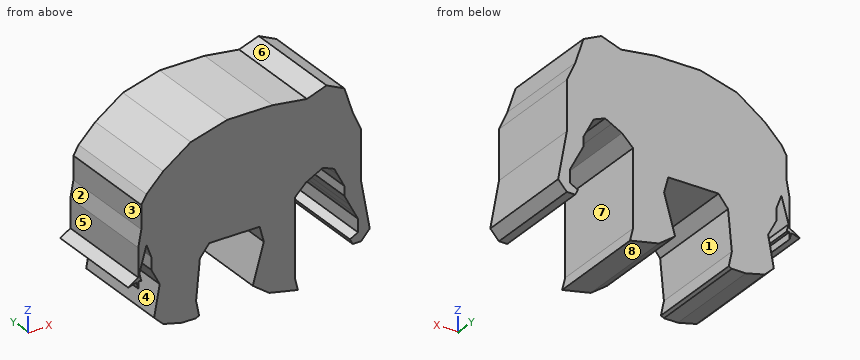
```python
from build123d import *

# Parameters (mm, degrees)
F1_DEPTH = 25.4


with BuildPart() as f1:
    # F0 (on Front) → F1 (new body)
    with BuildSketch(Plane.XZ):
        Polygon((19.687949, 25.243243), (14.781063, 23.544706), (6.194014, 24.701377), (-5.051399, 24.701377), (-14.188432, 22.223622), (-21.076944, 17.4111), (-25.228923, 13.259119), (-26.514801, 11.088767), (-26.514801, 5.281893), (-27.283788, 1.180633), (-27.283788, -5.896606), (-29.806441, -7.50078), (-27.718788, -6.934656), (-27.283788, -8.538775), (-27.283788, -6.790471), (-26.514801, -6.934656), (-27.021825, -5.06494), (-25.228923, 1.180633), (-24.035911, -2.027715), (-24.035911, -5.06494), (-21.926213, -9.104954), (-23.341661, -16.654009), (-21.076944, -18.824359), (-16.358785, -19.973479), (-12.867347, -19.973479), (-12.112442, -19.579267), (-12.867347, -15.899101), (-11.923715, -6.085332), (-9.564636, -3.160073), (2.985667, -3.160073), (4.023661, -7.028964), (1.287129, -16.654009), (5.344746, -19.579267), (12.516348, -21.089077), (11.761442, -17.975092), (11.761442, -16.654009), (11.761442, 1.08627), (14.527172, 3.790959), (17.145273, 5.158133), (18.744318, 5.993155), (21.584706, 4.860796), (22.52096, 3.067896), (24.123017, 0), (24.123017, -2.335592), (25.511982, -4.995424), (26.670383, -7.213729), (27.510151, -8.821864), (27.510151, -12.030212), (25.511982, -13.073657), (26.199007, -14.389291), (28.275, -14.389291), (30.445352, -12.030212), (28.275, 0), (28.275, 1.841175), (28.275, 4.860796), (28.275, 12.221124), (26.199007, 16.844919), (24.123017, 23.167253), align=None)
    extrude(amount=F1_DEPTH)


solid = f1.part
```
Geometry check sheet. Reference: the model listing, model coordinates, mm. Face numbers are marked on the shaded views. A direction names the side the tool comes from. Round coordinates to 2 decimals unless told otherwise and drop trailing zeros. Loops run counter-clockwise (first coordinate to the right, second up) from the corner with the lowest first, then second, coordinate; pieces in that order, holes last. Notation, with made-up numbers: (40.25, 42) - (47.25, 42) arc R29 ccw to (47.25, 62) - close; hole circle Ø3 at (8, 15). An arc over 180 degrees is marked (long way). Write item = value, one per line. Start each with the question number.
1. Section check C-C on x = -6. Enter the section's corners in (y, z), then the cut area to 3 significant figures.
2. Depth check by flat-ended pin: pin 1 (14 mm diameter, centred on x = -5.5, y = -11, fed in from -Z); pin 2 (10 mm diameter, centred on x = 16, y = -5, fed in from -Z); pin 3 (0.7 mm diameter, centred on y = -13.5, z = -1.5, fed in from -X). Enter the tip coordinate at first touch or a pass-through.
3. Section check A-A on z = -4. Enter the section's corners in (x, y), then the cut area to 3 significant figures.
4. Thickness scan on line 1 (X direction, y = -19, z = -10); line 2 (X direction, y = -11, z = -9); line 3 (X direction, y = -20.25, z = -6). Record the ranges inside material, lowest first.
5. Set-up check for the marked faces 4, 5, 6, 7 and 8: record each of +Z, -Z, +X, -X, +Y, -Y from which the full face is reachable in a straight line by a thin tool's end or side.
6. Mould release check, pull along Z, two halves, no side actions. Record for the marked faces 1, 2 and 3: released by +Z, released by -Z, zero draft, split by the parting line, or undercut.
7. Section check B-B on z = 2. Enter the section's corners in (x, y) (3 decimals).
8. Section check D-D on x = 7.5. Enter the section's corners in (y, z).
Working result:
q1.outline = (-25.4, -3.16) - (0, -3.16) - (0, 24.44) - (-25.4, 24.44) - close
q1.area = 701 mm^2
q2.pin_1 = -19.78
q2.pin_2 = -21.09
q2.pin_3 = -27.28
q3.outline = (-27.28, -25.4) - (-26.72, -25.4) - (-26.72, 0) - (-27.28, 0) - close; (-24.04, -25.4) - (-10.24, -25.4) - (-10.24, 0) - (-24.04, 0) - close; (3.21, -25.4) - (11.76, -25.4) - (11.76, 0) - (3.21, 0) - close; (24.99, -25.4) - (29, -25.4) - (29, 0) - (24.99, 0) - close
q3.area = 684 mm^2
q4.line_1 = -22.09 to -12.3, 3.18 to 11.76, 27.51 to 30.08
q4.line_2 = -21.98 to -12.2, 3.46 to 11.76, 27.51 to 29.9
q4.line_3 = -27.45 to -26.77, -23.55 to -11.85, 3.75 to 11.76, 26.04 to 29.36
q5.face_4 = -X, +Y, -Y
q5.face_5 = +Z, -X, +Y, -Y
q5.face_6 = +Z, +Y, -Y
q5.face_7 = +Y, -Y
q5.face_8 = -Z, +Y, -Y
q6.face_1 = undercut
q6.face_2 = released by +Z
q6.face_3 = zero draft
q7.outline = (-27.13, -25.4) - (12.696, -25.4) - (12.696, 0) - (-27.13, 0) - close; (23.079, -25.4) - (28.275, -25.4) - (28.275, 0) - (23.079, 0) - close
q8.outline = (-25.4, -20.03) - (0, -20.03) - (0, 24.53) - (-25.4, 24.53) - close
